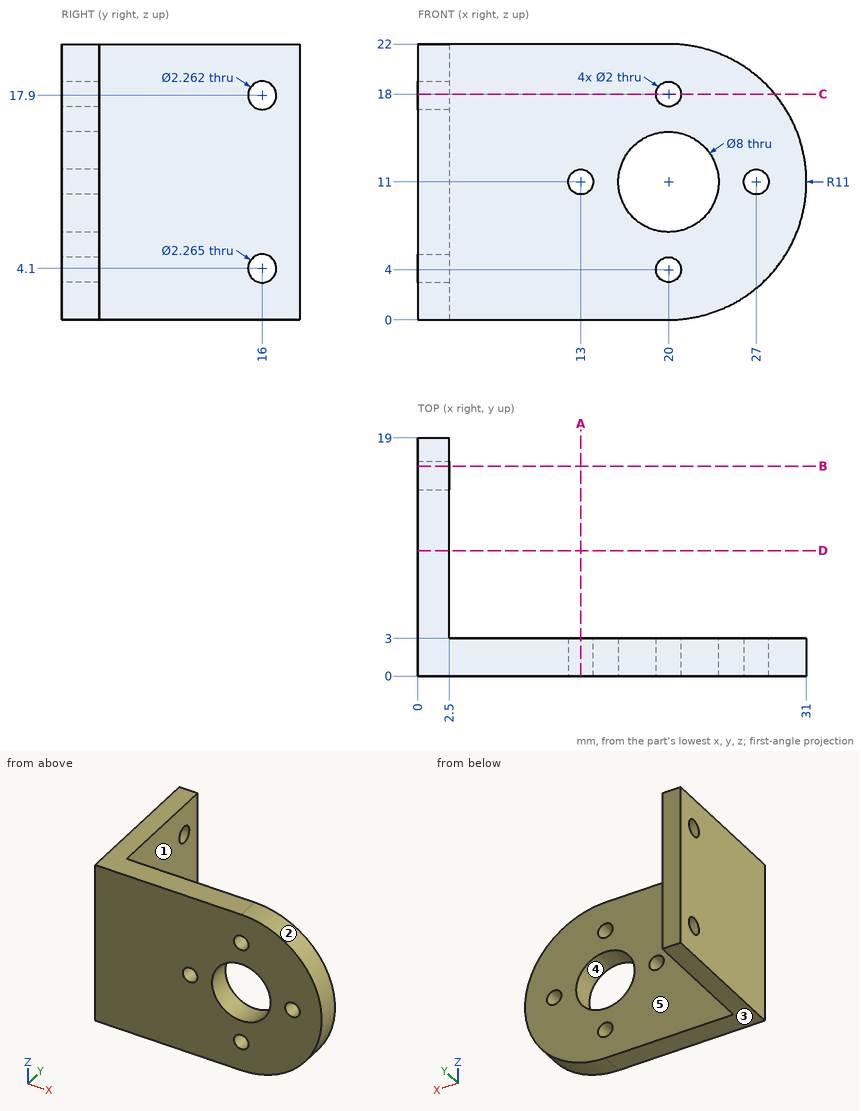
Part print with two shaded views. Sizes in mm from the minimum x, y, z corner. A direction names the side the tool comes from. Round coordinates to 2 decimals unless told otherwise and drop trailing zeros. Order: outer loops, then holes, each group sorted by start corner. A loop starts at its lowest first (then second) coordinate and runs counter-clockwise, first axis right, second up. Notation, with made-up numbers: (70, 14.5) -> (78, 14.5) arc R27 ccw to (78, 35.5) -> close; hole circle Ø3 at (82.25, 17). An arc over 180 degrees is marked (long way). Use one line per item in the form item = value.
Item 1: Cut at A-A, the plane x = 13. Write the cut outline in (y, z), and give its area (3 significant figures).
Returned:
outline = (0, 0) -> (3, 0) -> (3, 10) -> (0, 10) -> close; (0, 12) -> (3, 12) -> (3, 22) -> (0, 22) -> close
area = 60.0 mm^2
Item 2: Cut at B-B, the plane y = 16.75. Write the cut outline in (x, z).
Returned:
outline = (0, 0) -> (2.5, 0) -> (2.5, 3.25) -> (0, 3.25) -> close; (0, 4.95) -> (2.5, 4.95) -> (2.5, 17.05) -> (0, 17.05) -> close; (0, 18.75) -> (2.5, 18.75) -> (2.5, 22) -> (0, 22) -> close
Item 3: Drill centre lines: line 1 (X direction, y = 1.35, z = 11); line 2 (Z direction, x = 20, y = 1.1); line 3 (X direction, y = 1.25, z = 10.5). Where is each one in solid material? Low to high.
Returned:
line_1 = 0 to 12, 14 to 16, 24 to 26, 28 to 31
line_2 = 0 to 3, 5 to 7, 15 to 17, 19 to 22
line_3 = 0 to 12.13, 13.87 to 16.03, 23.97 to 26.13, 27.87 to 30.99
Item 4: Flat gauge pin, fed straight in: pin 1 Ø1 at (y, z) = (5, 5) entering from +X. Where does the tip first touch, or does it go through?
Returned:
pin_1 = 2.5
Item 5: Tool access for the marked faces 1 and 2: list every direction of +Z, -Z, +X, -X, +Y, -Y with a clear straight run to the whole face (end or side of a thin tool).
Returned:
face_1 = +Z, -Z, +X, +Y
face_2 = +X, +Y, -Y
Item 6: Cut at D-D, the plane y = 10. Write the cut outline in (x, z).
Returned:
outline = (0, 0) -> (2.5, 0) -> (2.5, 22) -> (0, 22) -> close
Item 7: Cut at C-C, the plane z = 18. Write the cut outline in (x, y) (1 decimal).
Returned:
outline = (0, 0) -> (19, 0) -> (19, 3) -> (2.5, 3) -> (2.5, 14.9) -> (0, 14.9) -> close; (0, 17.1) -> (2.5, 17.1) -> (2.5, 19) -> (0, 19) -> close; (21, 0) -> (28.5, 0) -> (28.5, 3) -> (21, 3) -> close
Item 8: Pull direction Z, two halves, no side cores. Call the marked faces 3, 4 and 5: released by +Z, released by -Z, zero draft, split by the parting line, or undercut.
Returned:
face_3 = released by -Z
face_4 = undercut
face_5 = zero draft
